Study the drawing (mm; zero at the part's minimum x, y, z) and answer. A direction names the side the tool comes from. Coordinates: 2 decimals unless noted, no trailing zeros. Loops run counter-clockwise (first coordinate to the right, second up) from the corner with the lowest first, then second, coordinate; pieces in that order, holes last. Notation, with made-up numbers: (86, 88) - (143, 88) arc R13 ccw to (143, 105) - close; hole circle Ø9 at (42, 45.5). An arc over 180 degrees is marked (long way). One line per item, written item: value. Start each with the question number.
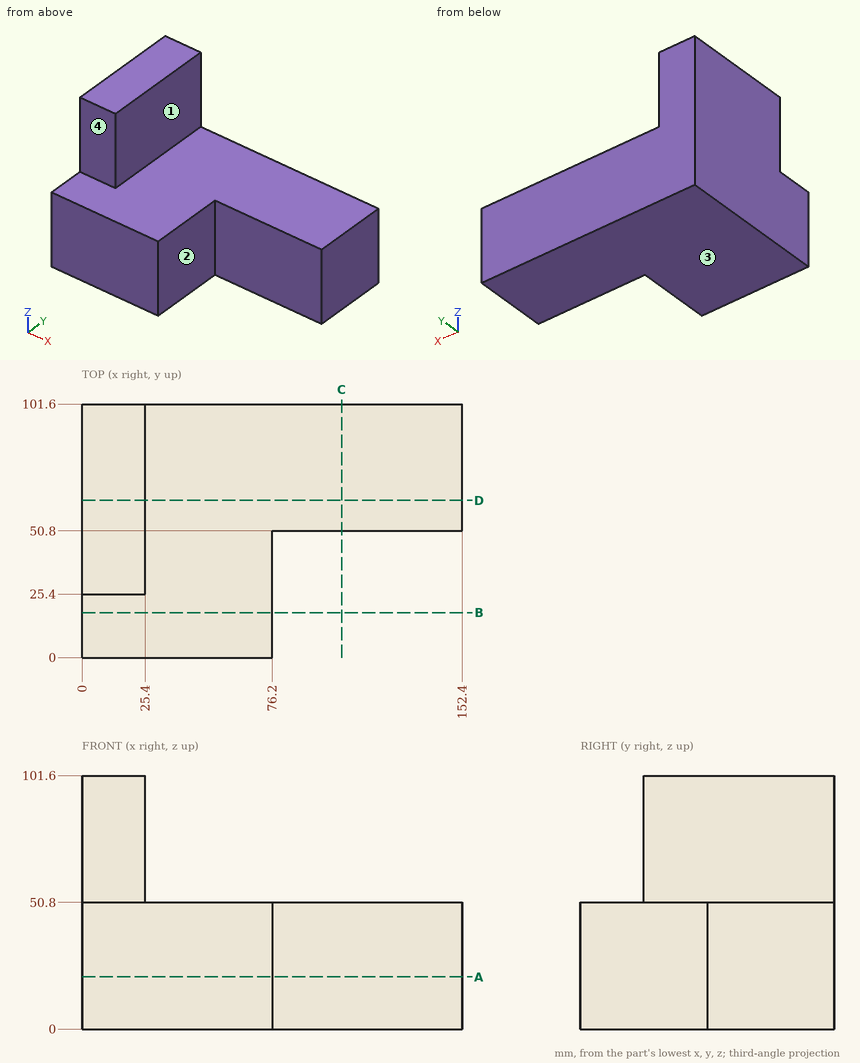
1) Flat-ended cylindrical pins translate along their axes: P1, Ø6, axis at x = 112.5, y = 52, coming from the +Z side; P2, Ø4, axis at y = 50, z = 65, coming from the +X side; P3, Ø1, axis at y = 38.5, z = 42, coming from the +X side. Find the tip coordinate at first contact, or state that the pin passes through.
2) Section A-A, the plane z = 21 is taken. Determine the outline of the cut face in (x, y).
3) Section C-C, the plane x = 104 is taken. Determine the outline of the cut face in (y, z), and give its area (3 significant figures).
4) Straight lines are drawn through the part: L1, parallel to Z at x = 141.5, y = 66; L2, parallel to X at y = 39.5, z = 85; L3, parallel to X at y = 39.5, z = 42.5. For each, find the intervals that lie inside material, in ascending order.
5) Section B-B, the plane y = 18 is taken. Determine the outline of the cut face in (x, z), and give its area (3 significant figures).
6) Section D-D, the plane y = 63 is taken. Determine the outline of the cut face in (x, z), and give its area (3 significant figures).
7) For the marked faces 1, 2, 3 and 4, determine the directions among +Z, -Z, +X, -X, +Y, -Y from which every point of the face is accessible in a straight line to the end or side of a thin tool.
Answer below:
1. P1: z = 50.8
1. P2: x = 25.4
1. P3: x = 76.2
2. outline: (0, 0) - (76.2, 0) - (76.2, 50.8) - (152.4, 50.8) - (152.4, 101.6) - (0, 101.6) - close
3. outline: (50.8, 0) - (101.6, 0) - (101.6, 50.8) - (50.8, 50.8) - close
3. area: 2,580 mm2
4. L1: 0 to 50.8
4. L2: 0 to 25.4
4. L3: 0 to 76.2
5. outline: (0, 0) - (76.2, 0) - (76.2, 50.8) - (0, 50.8) - close
5. area: 3,870 mm2
6. outline: (0, 0) - (152.4, 0) - (152.4, 50.8) - (25.4, 50.8) - (25.4, 101.6) - (0, 101.6) - close
6. area: 9,030 mm2
7. face 1: +Z, +X, +Y, -Y
7. face 2: +Z, -Z, +X, -Y
7. face 3: -Z, +X, -X, +Y, -Y
7. face 4: +Z, +X, -X, -Y
